```python
from build123d import *


with BuildPart() as part:
    # Croquis1 → Revolución2 (revolve)
    with BuildSketch(Plane(origin=(0, 0, 0), x_dir=(1, 0, 0), z_dir=(0, 1, 0)), mode=Mode.PRIVATE) as revoluci_n2_sk:
        Polygon((0, 4), (8, 4), (8, 5), (10, 5), (10, 9), (3, 9), (3, 7.5), (1, 7.5), (1, 9), (0.5, 9), (0, 8.5), align=None)
    revolve(revoluci_n2_sk.sketch.rotate(Axis((0, 0, 0), (1, 0, 0)), 180), axis=Axis((0, 0, 0), (1, 0, 0)))


solid = part.part
```
Geometry: final body of the model. Coordinates: model frame, mm. A direction names the side the tool comes from. Coordinates: 2 decimals unless noted, no trailing zeros. Order: outer loops, then holes, each group sorted by start corner. A loop starts at its lowest first (then second) coordinate and runs counter-clockwise, first axis right, second up. Notation, with made-up numbers: M 16,56 L 47,56 A17 ccw 47,71 Z; hole C -22,11.5 d2. An arc over 180 degrees is marked long. Answer in a Markdown table with one row per item. Add a question column.
Q1. Section query A-A on y = 0. Return the cut outline in (x, z), and give its area (4 significant figures).
Q2. Section query C-C on x = 7.5. Return the cut outline in (y, z).
Q3. Mould query, pull axis X, two halves, no side actions, for faces 4 (the flat face through (1, -7.4, 2)), 5 (the flat face through (10, 4, -4)), 6 (the cylindrical face through (4.056, 3.905, -0.867)). Classes: released by +X, released by -X, zero draft, split by the parting line, or undercut.
Q4. Reachability of faces 1 (the cylindrical face through (9, 0, -5)), 2 (the flat face through (0, 2, 4)), 3 (the cylindrical face through (1.986, -6.324, 4.032)) from +Z, -Z, +X, -X, +Y, -Y: full face, straight path, thin tool, end or side. Return the list, or none.
Q5. Line query: L1, parallel to Y at x = 9.25, z = 0; L2, parallel to Y at x = 4.75, z = 0; L3, parallel to X at y = 6.25, z = 5.5. Output: solid intervals per line, ascending.
Q6. Contact query for flat-ended pins moving along their axis: P1, Ø1, axis at x = 5.5, y = 3.5, coming from the -Z side; P2, Ø5, axis at x = 8, y = 7, coming from the -Z side; P3, Ø6, axis at x = 7.5, y = 4, coming from the -Z side. Output: stop coordinate, or through.
Completed:
| question | item | result |
|---|---|---|
| 1 | outline | M 0,-8.5 L 0.5,-9 L 1,-9 L 1,-7.5 L 3,-7.5 L 3,-9 L 10,-9 L 10,-5 L 8,-5 L 8,-4 L 0,-4 Z; M 0,4 L 8,4 L 8,5 L 10,5 L 10,9 L 3,9 L 3,7.5 L 1,7.5 L 1,9 L 0.5,9 L 0,8.5 Z |
| 1 | area | 89.75 mm2 |
| 2 | outline | C 0,0 d18; hole C 0,0 d8 |
| 3 | face 4 | undercut |
| 3 | face 5 | released by +X |
| 3 | face 6 | zero draft |
| 4 | face 1 | +X |
| 4 | face 2 | +Z, -Z, -X, +Y, -Y |
| 4 | face 3 | none |
| 5 | L1 | y = -9 to -5, 5 to 9 |
| 5 | L2 | y = -9 to -4, 4 to 9 |
| 5 | L3 | x = 0 to 1, 3 to 10 |
| 6 | P1 | stops at z = -8.49 |
| 6 | P2 | stops at z = -7.79 |
| 6 | P3 | stops at z = -8.94 |
